Can you work these out from the model? Positions are in its coordinate system, mm. A direction names the side the tool comes from. Give positions to 0.01 mm unless a question says otherwise; leave off trailing zeros. Loops run counter-clockwise (first coordinate to the right, second up) from the corner with the lowest first, then second, coordinate; pieces in that order, holes last. Notation, with made-up numbers: M 47,1.5 L 54,1.5 A25 cw 54,39.5 Z; hole C -25.75,73.5 d6. An arc over 180 degrees is marked long. Answer as a JSON object with one key per item and string values.
```python
from build123d import *

# Parameters (mm, degrees)
SKETCH1_W                                      = 127
SKETCH1_H                                      = 152.4
BOSS_EXTRUDE1_DEPTH                            = 12.7
SKETCH2_R                                      = 14.2875
CUT_EXTRUDE1_DEPTH                             = 13.7
SKETCH3_R                                      = 7.9375
SKETCH3_R_2                                    = 1.016
CUT_EXTRUDE2_DEPTH                             = 13.7
SKETCH4_R                                      = 36.195
CUT_EXTRUDE3_DEPTH                             = 6.35
SKETCH5_R                                      = 19.05
CUT_EXTRUDE4_DEPTH                             = 2.54
CSK_FOR_8_FLAT_HEAD_MACHINE_SCREW1_D           = 4.4958
CSK_FOR_8_FLAT_HEAD_MACHINE_SCREW1_CSINK_D     = 8.4328
CSK_FOR_8_FLAT_HEAD_MACHINE_SCREW1_CSINK_ANGLE = 82
FILLET1_R                                      = 12.7
SKETCH8_W                                      = 127
SKETCH8_H                                      = 3.175
BOSS_EXTRUDE2_DEPTH                            = 12.7
F_1_4_20_TAPPED_HOLE1_AT_2_COUNT               = 2
F_1_4_20_TAPPED_HOLE1_AT_2_PITCH               = 38.1
SKETCH11_W                                     = 12.7
SKETCH11_H                                     = 19.05
BOSS_EXTRUDE3_DEPTH                            = 12.7
SKETCH12_R                                     = 0.79375
CUT_EXTRUDE5_DEPTH                             = 13.7


with BuildPart() as part:
    # Sketch1 → Boss-Extrude1 (new body)
    with BuildSketch(Plane.XY):
        with Locations((0, 76.2)):
            Rectangle(SKETCH1_W, SKETCH1_H)
    extrude(amount=BOSS_EXTRUDE1_DEPTH)

    # Sketch2 → Cut-Extrude1 (cut, through all)
    with BuildSketch(Plane(origin=(0, 0, 0), x_dir=(-1, 0, 0), z_dir=(0, 0, -1))):
        with BuildLine():
            Line((44.45, 50.8), (63.5, 50.8))
            Line((63.5, 50.8), (63.5, 152.4))
            Line((63.5, 152.4), (-63.5, 152.4))
            Line((-63.5, 152.4), (-63.5, 50.8))
            Line((-63.5, 50.8), (-44.45, 50.8))
            Line((-44.45, 50.8), (-23.686198751, 104.421913036))
            ThreePointArc((-23.686198751, 104.421913036), (0, 120.65), (23.686198751, 104.421913036))
            Line((23.686198751, 104.421913036), (44.45, 50.8))
        make_face()
        with Locations((0, 95.25)):
            Circle(SKETCH2_R)
    extrude(amount=-CUT_EXTRUDE1_DEPTH, mode=Mode.SUBTRACT)

    # Sketch3 → Cut-Extrude2 (cut, through all)
    with BuildSketch(Plane.XY.offset(12.7)):
        with Locations((0, 44.45)):
            Circle(SKETCH3_R)
        with Locations((-25.019, 44.45)):
            Circle(SKETCH3_R_2)
        with Locations((25.019, 44.45)):
            Circle(SKETCH3_R_2)
        with Locations((0, 69.469)):
            Circle(SKETCH3_R_2)
        with Locations((0, 19.431)):
            Circle(SKETCH3_R_2)
    extrude(amount=-CUT_EXTRUDE2_DEPTH, mode=Mode.SUBTRACT)

    # Sketch4 → Cut-Extrude3 (cut)
    with BuildSketch(Plane.XY.offset(12.7)):
        with Locations((0, 44.45)):
            Circle(SKETCH4_R)
    extrude(amount=-CUT_EXTRUDE3_DEPTH, mode=Mode.SUBTRACT)

    # Sketch5 → Cut-Extrude4 (cut)
    with BuildSketch(Plane.XY.offset(6.35)):
        with Locations((0, 44.45)):
            Circle(SKETCH5_R)
    extrude(amount=-CUT_EXTRUDE4_DEPTH, mode=Mode.SUBTRACT)

    # CSK for _8 Flat Head Machine Screw1 (through all)
    with Locations(Plane(origin=(0, 0, 0), x_dir=(-1, 0, 0), z_dir=(0, 0, -1))):
        with Locations((0, 69.469), (25.019, 44.45), (0, 19.431), (-25.019, 44.45)):
            CounterSinkHole(CSK_FOR_8_FLAT_HEAD_MACHINE_SCREW1_D / 2, CSK_FOR_8_FLAT_HEAD_MACHINE_SCREW1_CSINK_D / 2, counter_sink_angle=CSK_FOR_8_FLAT_HEAD_MACHINE_SCREW1_CSINK_ANGLE)

    # Fillet1
    fillet1_edges = [part.edges().sort_by_distance(p)[0] for p in [
        (44.45, 50.8, 6.35),
        (-44.45, 50.8, 6.35),
    ]]
    fillet(fillet1_edges, radius=FILLET1_R)

    # Sketch8 → Boss-Extrude2 (add)
    with BuildSketch(Plane(origin=(0, 0, 0), x_dir=(-1, 0, 0), z_dir=(0, 0, -1))):
        with Locations((0, -1.5875)):
            Rectangle(SKETCH8_W, SKETCH8_H)
    extrude(amount=-BOSS_EXTRUDE2_DEPTH)

    # Sketch9 → 1_4-20 Tapped Hole1 (revolve, cut)
    with BuildSketch(Plane(origin=(63.5, 42.8625, 6.35), x_dir=(0, 0, -1), z_dir=(0, 1, 0))):
        Polygon((0, 0), (0, 18.043816902), (2.5527, 16.51), (2.5527, 0), align=None)
    f_1_4_20_tapped_hole1 = revolve(axis=Axis((69.85, 42.8625, 6.35), (-1, 0, 0)), mode=Mode.SUBTRACT)

    # 1_4-20 Tapped Hole1 at 2: 1_4-20 Tapped Hole1 ×2
    with Locations(*[(0, -i * F_1_4_20_TAPPED_HOLE1_AT_2_PITCH, 0) for i in range(1, F_1_4_20_TAPPED_HOLE1_AT_2_COUNT)]):
        add(f_1_4_20_tapped_hole1, mode=Mode.SUBTRACT)

    # Sketch11 → Boss-Extrude3 (add)
    with BuildSketch(Plane(origin=(63.5, 0, 0), x_dir=(0, 0, -1), z_dir=(1, 0, 0))):
        with Locations((-6.35, 23.8125)):
            Rectangle(SKETCH11_W, SKETCH11_H)
    boss_extrude3 = extrude(amount=BOSS_EXTRUDE3_DEPTH)

    # Sketch12 → Cut-Extrude5 (cut, through all)
    with BuildSketch(Plane.XY.offset(12.7)):
        with Locations((63.5, 34.13125)):
            Circle(SKETCH12_R)
        with Locations((63.5, 13.49375)):
            Circle(SKETCH12_R)
    cut_extrude5 = extrude(amount=-CUT_EXTRUDE5_DEPTH, mode=Mode.SUBTRACT)

    # Mirror1: Cut-Extrude5, Boss-Extrude3, 1_4-20 Tapped Hole1 across plane
    add(cut_extrude5.mirror(Plane(origin=(0, 0, 0), x_dir=(0, 0, 1), z_dir=(1, 0, 0))), mode=Mode.SUBTRACT)
    add(boss_extrude3.mirror(Plane(origin=(0, 0, 0), x_dir=(0, 0, 1), z_dir=(1, 0, 0))))
    add(f_1_4_20_tapped_hole1.mirror(Plane(origin=(0, 0, 0), x_dir=(0, 0, 1), z_dir=(1, 0, 0))), mode=Mode.SUBTRACT)

    # Mirror1 copy 1 sketch → Mirror1 copy 1 (revolve, cut)
    with BuildSketch(Plane(origin=(-63.5, 4.7625, 6.35), x_dir=(0, 0, -1), z_dir=(0, 1, 0))):
        Polygon((0, 0), (0, -18.043816902), (2.5527, -16.51), (2.5527, 0), align=None)
    revolve(axis=Axis((-69.85, 4.7625, 6.35), (-1, 0, 0)), mode=Mode.SUBTRACT)


solid = part.part
```
1) Suppose I cut it at D-D, the plane x = -34. Write out the boundary of the cut face in (y, z) (3 decimals), and give its area (3 significant figures).
Answer list:
{"outline": "M -3.175,0 L 77.787,0 L 77.787,12.7 L 56.863,12.7 L 56.863,6.35 L 32.037,6.35 L 32.037,12.7 L -3.175,12.7 Z", "area": "871 mm^2"}
2) Please list where these lines run through material, in increasing order: line 1 along Y through (x, z) = (-2.5, 8) (3 decimals); line 2 along X through (y, z) = (43, 4); line 3 along X through (y, z) = (43, 6.5). Write a range as from..to.
Answer list:
{"line 1": "-3.175..8.341, 80.559..81.183, 109.317..120.527", "line 2": "-46.87..-26.74, -23.3..-18.99, 18.99..23.3, 26.74..46.87", "line 3": "-45.58..-36.17, 36.17..45.58"}
3) For faces 1 (the cylindrical face through (-7.846, 9.116, 9.569)), 2 (the flat face through (-63.5, 42.8, 9.1)), 3 (the cylindrical face through (-55.361, 3.996, 3.915)), 4 (the flat face through (70, 14.288, 6)), which set-ups out of +Z, -Z, +X, -X, +Y, -Y let a thin tool reach every point of the face, with its end or its side?
Answer list:
{"face 1": "+Z", "face 2": "+Z, -Z, -X, +Y", "face 3": "-X", "face 4": "+Z, -Z, +X, -Y"}
4) Suppose I cut it at A-A, the plane z = 11. Give the number of separate pieces and of enclosed holes in the cut face, and give its area (3 significant figures).
Answer list:
{"separate pieces": "1", "enclosed holes": "2", "area": "6,820 mm^2"}
5) If we mould it in two halves opening along X, with no side actions, what happens to faces 5 (the flat face through (76.2, 24, 6)), 6 (the flat face through (16, 29, 6.35)), 7 (the cylindrical face through (-45.89, 53.08, 6.44))? For each: +X half, -X half, draft (parallel to the pull), parting line (faces both ways), or undercut.
Answer list:
{"face 5": "+X half", "face 6": "undercut", "face 7": "-X half"}
6) Suppose I cut it at B-B, the plane y = 95.25. Write out the boundary of the cut face in (x, z).
Answer list:
{"outline": "M -27.24,0 L -14.29,0 L -14.29,12.7 L -27.24,12.7 Z; M 14.29,0 L 27.24,0 L 27.24,12.7 L 14.29,12.7 Z"}
7) Will these pins go through, and if not, where does the flat tip stop? pin 1 Ø6 at (y, z) = (4.76, 6.35) entering from -X; pin 2 Ø2 at (y, z) = (13, 6.5) entering from +X; pin 3 Ø4 at (x, z) = (2, 7) entering from +Y; pin 4 Ø18.5 at (x, y) = (0, 44.45) entering from -Z.
Answer list:
{"pin 1": "x = -63.5", "pin 2": "x = 63.5", "pin 3": "y = 120.65", "pin 4": "z = 0"}
